Check sheet for the modelled part. Datum: model origin and axes. Units: mm. A direction names the side the tool comes from. Round coordinates to 2 decimals unless told otherwise and drop trailing zeros. Loops run counter-clockwise (first coordinate to the right, second up) from the corner with the lowest first, then second, coordinate; pieces in that order, holes last. Notation, with made-up numbers: (33.25, 41.25) -> (51.25, 41.25) arc R14 ccw to (51.25, 58.25) -> close; hole circle Ø7 at (-4.75, 73.5). An arc over 180 degrees is marked (long way). Return JSON: item names as keys, results as strings.
Autodesk Inventor part; units mm, degrees
ref_plane "YZ Plane" through (0, 0, 0) normal (1, 0, 0) x (0, 1, 0)
ref_plane "XZ Plane" through (0, 0, 0) normal (0, 1, 0) x (-1, 0, 0)
ref_plane "XY Plane" through (0, 0, 0) normal (0, 0, 1) x (1, 0, 0)
sketch "Эскиз2" plane through (0, 0, 0) normal (0, 0, 1) x (1, 0, 0)
  line L0 (-5, -5) -> (5, -5)
  line L1 (6, -4) -> (6, 4)
  line L2 (5, 5) -> (-5, 5)
  line L3 (-6, 4) -> (-6, -4)
  line L4 (-6, -5) -> (6, 5) construction
  line L5 (6, -5) -> (-6, 5) construction
  arc A0 (-5, 5) -> (-6, 4) centre (-5, 4) ccw
  arc A1 (6, 4) -> (5, 5) centre (5, 4) ccw
  arc A2 (5, -5) -> (6, -4) centre (5, -4) ccw
  arc A3 (-6, -4) -> (-5, -5) centre (-5, -4) ccw
  arc A4 (-3.3166, 5) -> (-3.3166, -5) centre (0, 0) ccw
  arc A5 (3.3166, -5) -> (3.3166, 5) centre (0, 0) ccw
  dimension "d0" = 12
  dimension "d1" = 10
  dimension "d2" = 1
extrude "Выдавливание1" add sketch "Эскиз2" against normal blind 15 contours A4 L2 A5 L0
extrude "Выдавливание2" add sketch "Эскиз2" along normal blind 9
sketch "Эскиз3" plane through (0, 0, 9) normal (0, 0, 1) x (1, 0, 0)
  arc A0 (-1.118, 1) -> (1.118, 1) centre (0, 0) ccw
  circle A1 centre (0, 0) radius 2
  line L0 (-1.118, 1) -> (1.118, 1)
  arc A2 (1.118, 1) -> (-1.118, 1) centre (0, 0) ccw construction
  dimension "d8" = 3
  dimension "d9" = 4
  dimension "d10" = 2.5
extrude "Выдавливание3" add sketch "Эскиз3" along normal blind 1 contours L0 A0 | A1
extrude "Выдавливание4" add sketch "Эскиз3" along normal blind 10 contours L0 A0
sketch "Эскиз4" plane through (0, 0, -15) normal (0, 0, -1) x (-1, 0, 0)
  circle A0 centre (0, 0) radius 2.5
  line L0 (-4, 0.75) -> (-3.5, 0.75)
  line L1 (-3.5, 0.75) -> (-3.5, -0.75)
  line L2 (-3.5, -0.75) -> (-4, -0.75)
  line L3 (-4, -0.75) -> (-4, 0.75)
  line L4 (3.5, 0.75) -> (4, 0.75)
  line L5 (4, 0.75) -> (4, -0.75)
  line L6 (4, -0.75) -> (3.5, -0.75)
  line L7 (3.5, -0.75) -> (3.5, 0.75)
  line L8 (-3.5, 0) -> (3.5, 0) construction
  dimension "d15" = 5
  dimension "d18" = 8
  dimension "d19" = 7
  dimension "d20" = 1.5
extrude "Выдавливание5" add sketch "Эскиз4" along normal blind 1.75 contours A0
extrude "Выдавливание6" add sketch "Эскиз4" along normal blind 2.25 contours L0 L1 L2 L3 | L4 L5 L6 L7
fillet "Сопряжение1" radius 0.75 4 edges at (3.75, 0.75, -17.25) (3.75, -0.75, -17.25) (-3.75, 0.75, -17.25) (-3.75, -0.75, -17.25)
properties part number "Мотор 15x12x10 с редуктоом"
Q1. Material ranges on line 1 (Z direction, x = -4.25, y = 2.25); line 2 (Y direction, x = 5, z = -14); line 3 (Z direction, x = -1.25, y = 0), recorded low to high.
Results list:
{"line 1": "-15 to 9", "line 2": "-3.32 to 3.32", "line 3": "-16.75 to 19"}
Q2. Section check C-C (z = -0.5). Record the boundary of the cut face in (x, y), then the cut area to 3 significant figures.
Results list:
{"outline": "(-3.32, -5) -> (3.32, -5) arc R6 ccw to (3.32, 5) -> (-3.32, 5) arc R6 ccw to start", "area": "104 mm^2"}
Q3. Tool access check on faces 1 (the cylindrical face through (6, 0, -7)), 2 (the cylindrical face through (-6, 0, -7)), 3 (the flat face through (0, 1, 14)). Record the directions out of +Z, -Z, +X, -X, +Y, -Y that give a thin tool (end or side, any length) a straight path to the whole face; none if there is none.
Results list:
{"face 1": "-Z, +X", "face 2": "-Z, -X", "face 3": "+Z, +X, -X, +Y"}
Q4. Draft check along X on faces 4 (the flat face through (0, -5, -3)), 5 (the flat face through (0, 0, -16.75)), 6 (the flat face through (4, 0, -16)). Enter one of: released by +X, released by -X, zero draft, split by the parting line, or undercut.
Results list:
{"face 4": "zero draft", "face 5": "undercut", "face 6": "released by +X"}
Q5. Section check A-A (x = 0). Record the boundary of the cut face in (y, z).
Results list:
{"outline": "(-5, -15) -> (-2.5, -15) -> (-2.5, -16.75) -> (2.5, -16.75) -> (2.5, -15) -> (5, -15) -> (5, 9) -> (2, 9) -> (2, 10) -> (1, 10) -> (1, 19) -> (-1.5, 19) -> (-1.5, 10) -> (-2, 10) -> (-2, 9) -> (-5, 9) -> close"}
Q6. Section check D-D (y = -3.25). Record the boundary of the cut face in (x, z).
Results list:
{"outline": "(-6, 0) -> (-5.04, 0) -> (-5.04, -15) -> (5.04, -15) -> (5.04, 0) -> (6, 0) -> (6, 9) -> (-6, 9) -> close"}
Q7. Section check B-B (y = 1.5). Record the boundary of the cut face in (x, z).
Results list:
{"outline": "(-6, 0) -> (-5.81, 0) -> (-5.81, -15) -> (-2, -15) -> (-2, -16.75) -> (2, -16.75) -> (2, -15) -> (5.81, -15) -> (5.81, 0) -> (6, 0) -> (6, 9) -> (1.32, 9) -> (1.32, 10) -> (-1.32, 10) -> (-1.32, 9) -> (-6, 9) -> close"}
Q8. Go/stop test with flat-tipped pins: pin 1 (0.8 mm diameter, centred on y = 0.5, z = -16, fed in from -X); pin 2 (0.7 mm diameter, centred on x = 0.5, z = 13.5, fed in from +Y); pin 3 (1.5 mm diameter, centred on x = -4.5, z = 11.5, fed in from -Y); pin 4 (3 mm diameter, centred on x = 5, y = 3.5, fed in from -Z). Record where each tip stops, or that it passes through.
Results list:
{"pin 1": "x = -4", "pin 2": "y = 1", "pin 3": "through", "pin 4": "z = -15"}
